from build123d import *

# Parameters (mm, degrees)
F1_DEPTH = 38.1
F3_DEPTH = 12.7
F5_DEPTH = 12.7


with BuildPart() as f1:
    # F0 (on Front) → F1 (new body)
    with BuildSketch(Plane.XZ):
        Polygon((0, 63.183765), (-44.45, 63.639142), (-44.45, 31.889142), (12.7, 31.889142), align=None)
    extrude(amount=F1_DEPTH)

    # F2 (on face) → F3 (cut)
    with BuildSketch(Plane.XZ.offset(38.1)):
        Polygon((0, 63.183765), (-25.4, 63.443981), (-12.7, 31.889142), (12.7, 31.889142), align=None)
    extrude(amount=-F3_DEPTH, mode=Mode.SUBTRACT)

    # F4 (on face) → F5 (cut)
    with BuildSketch(Plane(origin=(0, 0, 0), x_dir=(-1, 0, 0), z_dir=(0, 1, 0))):
        Polygon((12.7, 31.889142), (25.4, 63.443981), (0, 63.183765), (-12.7, 31.889142), align=None)
    extrude(amount=-F5_DEPTH, mode=Mode.SUBTRACT)


solid = f1.part
Here's how the part is built. I have some questions about the finished solid (model axes, mm). A direction names the side the tool comes from. Coordinates: 2 decimals unless noted, no trailing zeros. Order: outer loops, then holes, each group sorted by start corner. A loop starts at its lowest first (then second) coordinate and runs counter-clockwise, first axis right, second up. Notation, with made-up numbers: M 22.5,15.25 L 31.5,15.25 A19 cw 31.5,43.25 Z; hole C -17.75,0 d6. An arc over 180 degrees is marked long. Answer as CSV lines item,"result". Start each with the question number.
1. I want a section at A-A, the plane z = 61. Write out the boundary of the cut face in (x, y), and give its area (3 significant figures).
2. For pin 1 (6 mm diameter, centred on x = -21.5, z = 57, fed in from +Y); pin 2 (10 mm diameter, centred on x = -31.5, y = -33.5, fed in from +Z); pin 3 (3 mm diameter, centred on x = -4.5, z = 35.5, fed in from +Y); pin 4 (4 mm diameter, centred on x = -24.5, y = -23, fed in from +Z), each with a flat end and sliding along its axis, tell me the tip position at first contact or that it passes through.
3. I want a section at D-D, the plane z = 43. Write out the boundary of the cut face in (x, y), and give its area (3 significant figures).
4. I need wall thicknesses on line 1 (Y direction, x = -15, z = 39.5); line 2 (Z direction, x = -29, y = -29); line 3 (X direction, y = -10, z = 53). Which ranges of each line are inside material? Lowest first, please. Write a range as [from, to].
5. I want a section at C-C, the plane x = 9. Write out the boundary of the cut face in (y, z), and give its area (3 significant figures).
6. I want a section at B-B, the plane y = -35.5. Write out the boundary of the cut face in (x, z), and give its area (3 significant figures).
7. On a 3-axis mill with a long thin cutter (end or side, diameter ignored), from which of +Z, -Z, +X, -X, +Y, -Y can I reach the whole of each face in a straight line? I mean faces 1 (the flat face through (-23, -19, 31.889)), 2 (the flat face through (-6, -12.7, 48)), 3 (the flat face through (-7, -25.4, 48)). Say none if no direction works.
Recorded:
1,outline,"M -44.45,-38.1 L -24.42,-38.1 L -24.42,-25.4 L 0.89,-25.4 L 0.89,-12.7 L -24.42,-12.7 L -24.42,0 L -44.45,0 Z"
1,area,"1,080 mm2"
2,pin 1,"stops at y = 0"
2,pin 2,"stops at z = 63.56"
2,pin 3,"stops at y = -12.7"
2,pin 4,"stops at z = 63.46"
3,outline,"M -44.45,-38.1 L -17.17,-38.1 L -17.17,-25.4 L 8.19,-25.4 L 8.19,-12.7 L -17.17,-12.7 L -17.17,0 L -44.45,0 Z"
3,area,"1,360 mm2"
4,line 1,"y = [-25.4, -12.7]"
4,line 2,"z = [31.89, 63.48]"
4,line 3,"x = [-44.45, -21.2]"
5,outline,"M -25.4,31.89 L -12.7,31.89 L -12.7,41.01 L -25.4,41.01 Z"
5,area,"116 mm2"
6,outline,"M -44.45,31.89 L -12.7,31.89 L -25.4,63.44 L -44.45,63.64 Z"
6,area,"803 mm2"
7,face 1,"-Z, +X, -X, +Y, -Y"
7,face 2,"+Z, +X, +Y"
7,face 3,"+Z, +X, -Y"
